```python
from build123d import *

# Parameters (mm, degrees)
SKETCH1_W           = 50
SKETCH1_H           = 50
SKETCH1_R           = 5
SKETCH1_R_2         = 1.666
SKETCH1_R_3         = 1.793902259
BOSS_EXTRUDE3_DEPTH = 10
SKETCH2_W           = 50
SKETCH2_H           = 10
BOSS_EXTRUDE4_DEPTH = 10
SKETCH3_W           = 50
SKETCH3_H           = 10
BOSS_EXTRUDE5_DEPTH = 30
SKETCH4_R           = 1.666
CUT_EXTRUDE1_DEPTH  = 30


with BuildPart() as part:
    # Sketch1 → Boss-Extrude3 (new body)
    with BuildSketch(Plane(origin=(0, 0, 0), x_dir=(1, 0, 0), z_dir=(0, 1, 0))):
        Rectangle(SKETCH1_W, SKETCH1_H)
        Circle(SKETCH1_R, mode=Mode.SUBTRACT)
        with Locations((-17, 17)):
            Circle(SKETCH1_R_2, mode=Mode.SUBTRACT)
        with Locations((17, 17)):
            Circle(SKETCH1_R_2, mode=Mode.SUBTRACT)
        with Locations((-17, -17)):
            Circle(SKETCH1_R_2, mode=Mode.SUBTRACT)
        with Locations((17, -19.536960904)):
            Circle(SKETCH1_R_3, mode=Mode.SUBTRACT)
    extrude(amount=BOSS_EXTRUDE3_DEPTH)

    # Sketch2 → Boss-Extrude4 (add)
    with BuildSketch(Plane(origin=(0, 0, -25), x_dir=(-1, 0, 0), z_dir=(0, 0, -1))):
        with Locations((0, 5)):
            Rectangle(SKETCH2_W, SKETCH2_H)
    extrude(amount=BOSS_EXTRUDE4_DEPTH)

    # Sketch3 → Boss-Extrude5 (add)
    with BuildSketch(Plane(origin=(0, 0, 0), x_dir=(-1, 0, 0), z_dir=(0, -1, 0))):
        with Locations((0, 30)):
            Rectangle(SKETCH3_W, SKETCH3_H)
    extrude(amount=BOSS_EXTRUDE5_DEPTH)

    # Sketch4 → Cut-Extrude1 (cut)
    with BuildSketch(Plane.XY.offset(-25)):
        with Locations((17, -22)):
            Circle(SKETCH4_R)
        with Locations((0, -10)):
            Circle(SKETCH4_R)
        with Locations((-17, -22)):
            Circle(SKETCH4_R)
    extrude(amount=-CUT_EXTRUDE1_DEPTH, mode=Mode.SUBTRACT)


solid = part.part
```
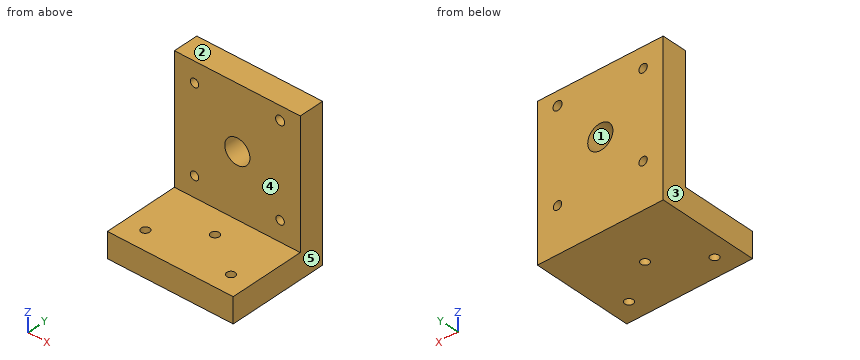
Read the model definition and answer for the solid it produces. Units are mm, in the model's axes. Face numbers are marked on the shaded views. A direction names the side the tool comes from. Give positions to 0.01 mm unless a question says otherwise; leave off trailing zeros. Write each loop counter-clockwise with the first axis right and the second up, starting at its lowest first coordinate (ties: lowest second). Pieces come first, ordered by that corner, then holes. Notation, with made-up numbers: (-19.5, 51.5) -> (36.5, 51.5) arc R12 ccw to (36.5, 55.5) -> close; hole circle Ø10 at (-12.5, 29.5). An arc over 180 degrees is marked (long way). Answer in a Markdown table with one row per item.
1) Straight lines are drawn through the part: line 1 (Z direction, x = 17, y = 6); line 2 (X direction, y = 3, z = -17); line 3 (Z direction, x = -17, y = 2). For each, find the intervals that lie inside material, in ascending order. Write a range as [from, to].
Results list:
| item | result |
|---|---|
| line 1 | [-35, -18.67], [-15.33, 17.74], [21.33, 25] |
| line 2 | [-25, -18.67], [-15.33, 15.33], [18.67, 25] |
| line 3 | [-35, -18.67], [-15.33, 15.33], [18.67, 25] |
2) Each of these flat-tipped pins is pushed along its axis until it touches: pin 1 Ø4 at (x, z) = (17, -17) entering from -Y; pin 2 Ø5.5 at (x, y) = (17, -22) entering from +Z; pin 3 Ø4 at (y, z) = (-3, 11.5) entering from +X. Where does it stop, or does it pass through?
Results list:
| item | result |
|---|---|
| pin 1 | y = 0 |
| pin 2 | z = -25 |
| pin 3 | through |
3) A tool of negligible diameter and unlimited length cuts with its end or side. For the marked faces 4 and 5, from which of +Z, -Z, +X, -X, +Y, -Y can it reach the whole face along a straight path? Write none if from no direction.
Results list:
| item | result |
|---|---|
| face 4 | +Z, +X, -X, -Y |
| face 5 | +Z, -Z, +X, +Y, -Y |
4) Section A-A on x = 3 is taken. Give the vertices of the cut face in (y, z).
Results list:
| item | result |
|---|---|
| outline | (-30, -35) -> (10, -35) -> (10, -4) -> (0, -4) -> (0, -25) -> (-30, -25) -> close; (0, 4) -> (10, 4) -> (10, 25) -> (0, 25) -> close |
5) Section B-B on z = 0 is taken. Give the vertices of the cut face in (x, y).
Results list:
| item | result |
|---|---|
| outline | (-25, 0) -> (-5, 0) -> (-5, 10) -> (-25, 10) -> close; (5, 0) -> (25, 0) -> (25, 10) -> (5, 10) -> close |
6) Section C-C on y = -22 is taken. Give the vertices of the cut face in (x, z), plus the area to 3 significant figures.
Results list:
| item | result |
|---|---|
| outline | (-25, -35) -> (-18.67, -35) -> (-18.67, -25) -> (-25, -25) -> close; (-15.33, -35) -> (15.33, -35) -> (15.33, -25) -> (-15.33, -25) -> close; (18.67, -35) -> (25, -35) -> (25, -25) -> (18.67, -25) -> close |
| area | 433 mm^2 |
7) Determine the mould class of the marked faces 1, 2 and 3 for opening direction X: released by +X, released by -X, zero draft, split by the parting line, or undercut.
Results list:
| item | result |
|---|---|
| face 1 | undercut |
| face 2 | zero draft |
| face 3 | released by -X |
8) Section D-D on x = 17 is taken. Give the vertices of the cut face in (y, z), plus the area to 3 significant figures.
Results list:
| item | result |
|---|---|
| outline | (-30, -35) -> (-23.67, -35) -> (-23.67, -25) -> (-30, -25) -> close; (-20.33, -35) -> (10, -35) -> (10, -18.67) -> (0, -18.67) -> (0, -25) -> (-20.33, -25) -> close; (0, -15.33) -> (10, -15.33) -> (10, 17.74) -> (0, 17.74) -> close; (0, 21.33) -> (10, 21.33) -> (10, 25) -> (0, 25) -> close |
| area | 797 mm^2 |
